Design review of the part built by this model. Coordinates are the model's own, in mm. Round coordinates to 2 decimals unless told otherwise and drop trailing zeros. Order: outer loops, then holes, each group sorted by start corner. A loop starts at its lowest first (then second) coordinate and runs counter-clockwise, first axis right, second up. Notation, with made-up numbers: (51.25, -24) - (56.25, -24) arc R24 ccw to (56.25, 4) - close; hole circle Ø4 at (-20, 43). An arc over 180 degrees is marked (long way). Answer as a JSON object with one key per item and string values. Group by question number.
Autodesk Inventor part; units mm, degrees
ref_plane "YZ Plane" through (0, 0, 0) normal (1, 0, 0) x (0, 1, 0)
ref_plane "XZ Plane" through (0, 0, 0) normal (0, 1, 0) x (-1, 0, 0)
ref_plane "XY Plane" through (0, 0, 0) normal (0, 0, 1) x (1, 0, 0)
sketch "Sketch1" plane through (0, 0, 0) normal (0, 0, 1) x (1, 0, 0)
  line L0 (-35.5, 21.8) -> (35.5, 21.8)
  line L1 (35.5, 21.8) -> (35.5, -21.8)
  line L2 (35.5, -21.8) -> (-35.5, -21.8)
  line L3 (-35.5, -21.8) -> (-35.5, 21.8)
  line L4 (-6.5, 21.8) -> (6.5, 21.8)
  line L5 (6.5, 21.8) -> (6.5, 20.3)
  line L6 (6.5, 20.3) -> (-6.5, 20.3)
  line L7 (-6.5, 20.3) -> (-6.5, 21.8)
  line L8 (-33.5, 19.75) -> (33.5, 19.75) construction
  line L9 (33.5, 19.75) -> (33.5, -19.75) construction
  line L10 (33.5, -19.75) -> (-33.5, -19.75) construction
  line L11 (-33.5, -19.75) -> (-33.5, 19.75) construction
  point P0 (0, 0)
  point P1 (0, 21.8)
  point P2 (35.5, 0)
  point P3 (0, 20.3)
  point P4 (33.5, 0)
  point P5 (0, -19.75)
  dimension "d0" = 43.6
  dimension "d1" = 71
  dimension "d2" = 13
  dimension "d3" = 1.5
  dimension "d4" = 67
  dimension "d5" = 39.5
extrude "Extrusion1" add sketch "Sketch1" along normal blind 1 contours L0 L7 L6 L5 L1 L2 L3
hole "Hole1" at (-33.5, 19.75, 0) at (33.5, 19.75, 0) at (33.5, -19.75, 0) at (-33.5, -19.75, 0) direction (0, 0, 1) diameter 2.4 end through all
properties part number "oled2.42-pcb"
1. Take a section at B-B, the plane y = -19.75. Give the boundary of the cut face in (x, z).
2. Clearance check with a flat-ended pin moving along its axis: P1, Ø0.5, axis at x = -1.5, z = 0.5, coming from the +Y side. State where the tip first meets the part, or that it passes through.
3. To check wall thickness, follow line 1 (X direction, y = 19.75, z = 0.7); line 2 (Y direction, x = 33.5, z = 0.35); line 3 (Y direction, x = -4, z = 0.2). State the ranges of each line that lie inside material, in increasing order. Write a range as from..to.
4. Mouldability with a two-part tool opening along Y and no side actions: class faces 1 (the cylindrical face through (32.31, 19.59, 0.51)), 2 (the cylindrical face through (-34.69, -19.91, 0.51)), 3 (the flat face through (0, 0, 0)) as pulls with the +Y half, pulls with the -Y half, needs draft (parallel to the pull), parting line crosses it, or undercut.
5. Take a section at A-A, the plane x = 33.5. Give the boundary of the cut face in (y, z), then the cut area to 3 significant figures.
Response values:
{
 "1": {"outline": "(-35.5, 0) - (-34.7, 0) - (-34.7, 1) - (-35.5, 1) - close; (-32.3, 0) - (32.3, 0) - (32.3, 1) - (-32.3, 1) - close; (34.7, 0) - (35.5, 0) - (35.5, 1) - (34.7, 1) - close"},
 "2": {"P1": "y = 20.3"},
 "3": {"line 1": "-35.5..-34.7, -32.3..32.3, 34.7..35.5", "line 2": "-21.8..-20.95, -18.55..18.55, 20.95..21.8", "line 3": "-21.8..20.3"},
 "4": {"face 1": "undercut", "face 2": "undercut", "face 3": "needs draft"},
 "5": {"outline": "(-21.8, 0) - (-20.95, 0) - (-20.95, 1) - (-21.8, 1) - close; (-18.55, 0) - (18.55, 0) - (18.55, 1) - (-18.55, 1) - close; (20.95, 0) - (21.8, 0) - (21.8, 1) - (20.95, 1) - close", "area": "38.8 mm2"}
}
